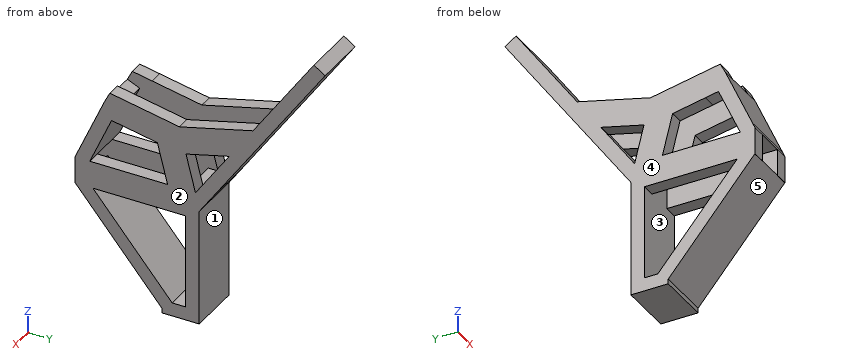
```python
from build123d import *

# Parameters (mm, degrees)
SKETCH_1_W       = 160
SKETCH_1_H       = 40
EXTRUDE_1_DEPTH  = 400
EXTRUDE_6_DEPTH  = 160
SKETCH_11_W      = 40
SKETCH_11_H      = 40
EXTRUDE_7_DEPTH  = 160
EXTRUDE_11_DEPTH = 160
SKETCH_17_W      = 40
SKETCH_17_H      = 80
EXTRUDE_13_DEPTH = 328
EXTRUDE_17_DEPTH = 160
EXTRUDE_18_DEPTH = 40
SKETCH_29_W      = 40
SKETCH_29_H      = 210
EXTRUDE_19_DEPTH = 80
EXTRUDE_20_DEPTH = 40
EXTRUDE_21_DEPTH = 40
EXTRUDE_22_DEPTH = 40


with BuildPart() as part:
    # Эскиз1 → Бобышка-Вытянуть1 (new body)
    with BuildSketch(Plane.XY):
        with Locations((41.709401709, 20)):
            Rectangle(SKETCH_1_W, SKETCH_1_H)
    extrude(amount=EXTRUDE_1_DEPTH)

    # Эскиз8 → Бобышка-Вытянуть6 (add)
    with BuildSketch(Plane.ZY.offset(38.290598291)):
        Polygon((403.40525509, 80.13918018), (346.080564925, 40), (400, 40), (400, 28.923811345), (901.472451167, 380.058601857), (878.529393713, 412.824683628), align=None)
    extrude(amount=-EXTRUDE_6_DEPTH)

    # Эскиз11 → Бобышка-Вытянуть7 (add)
    with BuildSketch(Plane.ZY.offset(38.290598291)):
        with Locations((20, -20)):
            Rectangle(SKETCH_11_W, SKETCH_11_H)
    extrude(amount=-EXTRUDE_7_DEPTH)

    # Эскиз12 → Бобышка-Вытянуть11 (add)
    with BuildSketch(Plane.ZY.offset(38.290598291)):
        Polygon((346.417777248, -297.115043875), (40, -40), (0, -40), (0, -70.641777725), (14.288495613, -70.641777725), (320.70627286, -327.756821599), align=None)
    extrude(amount=-EXTRUDE_11_DEPTH)

    # Эскиз17 → Бобышка-Вытянуть13 (add)
    with BuildSketch(Plane(origin=(0, 0, 0), x_dir=(-1, 0, 0), z_dir=(0, -1, 0))):
        with Locations((18.290598291, -360)):
            Rectangle(SKETCH_17_W, SKETCH_17_H)
        with Locations((-101.709401709, -360)):
            Rectangle(SKETCH_17_W, SKETCH_17_H)
    extrude(amount=EXTRUDE_13_DEPTH)

    # Эскиз26 → Бобышка-Вытянуть17 (add)
    with BuildSketch(Plane.ZY.offset(38.290598291)):
        Polygon((400, -284.21454886), (400, -328), (416.269465723, -320.756367165), align=None)
        Polygon((582.709091529, -202.867220245), (598.978557252, -239.40903855), (416.269465723, -320.756367165), (400, -284.21454886), align=None)
    extrude(amount=-EXTRUDE_17_DEPTH)

    # Эскиз27 → Бобышка-Вытянуть18 (add)
    with BuildSketch(Plane.ZY.offset(38.290598291)):
        Polygon((509.482462661, -33.639974138), (588.04709667, -18.55361331), (616.334023223, -165.862302077), (537.769389214, -180.948662905), align=None)
        Polygon((545.18630579, -219.573440808), (582.709091529, -202.867220245), (595.238756951, -231.009309548), (627.648793843, -224.785777584), (616.334023223, -165.862302077), (537.769389214, -180.948662905), align=None)
        Polygon((627.648793843, -224.785777584), (595.238756951, -231.009309548), (598.978557252, -239.40903855), align=None)
    extrude(amount=-EXTRUDE_18_DEPTH)

    # Эскиз29 → Бобышка-Вытянуть19 (add)
    with BuildSketch(Plane(origin=(0, 108.244163778, 563.698774535), x_dir=(1, 0, 0), z_dir=(0, 0.18857951034822912, 0.9820579251127819))):
        with Locations((101.709401709, -234.114356543)):
            Rectangle(SKETCH_29_W, SKETCH_29_H)
    extrude(amount=-EXTRUDE_19_DEPTH)

    # Эскиз33 → Бобышка-Вытянуть20 (add)
    with BuildSketch(Plane(origin=(121.709401709, 0, 0), x_dir=(0, 0, -1), z_dir=(1, 0, 0))):
        Polygon((-627.648793843, -224.785777584), (-598.978557252, -239.40903855), (-595.238756951, -231.009309548), align=None)
    extrude(amount=-EXTRUDE_20_DEPTH)

    # Эскиз34 → Бобышка-Вытянуть21 (add)
    with BuildSketch(Plane.ZY.offset(38.290598291)):
        Polygon((400, -53.586571178), (490.897529352, -76.536037974), (510.481100679, 1.029958017), (400, 28.923811345), align=None)
        Polygon((510.481100679, 1.029958017), (490.897529352, -76.536037974), (514.961644961, -62.173691245), (509.482462661, -33.639974138), (588.04709667, -18.55361331), align=None)
        Polygon((514.961644961, -62.173691245), (490.897529352, -76.536037974), (519.0862075, -83.653009555), align=None)
        Polygon((542.761910091, 128.886776961), (510.481100679, 1.029958017), (588.04709667, -18.55361331), (642.991448698, 199.068255444), align=None)
    extrude(amount=-EXTRUDE_21_DEPTH)

    # Эскиз35 → Бобышка-Вытянуть22 (add)
    with BuildSketch(Plane(origin=(121.709401709, 0, 0), x_dir=(0, 0, -1), z_dir=(1, 0, 0))):
        Polygon((-588.04709667, -18.55361331), (-643.423626769, 199.370869787), (-543.015704436, 129.064485674), (-510.437956524, 0.860554126), (-400, 28.923811345), (-400, -53.618639699), (-519.131929063, -83.891111895), (-509.482462661, -33.639974138), align=None)
    extrude(amount=-EXTRUDE_22_DEPTH)


solid = part.part
```
Could you check a few things on this model? Use its own coordinates, in mm. Face numbers are marked on the shaded views. A direction names the side the tool comes from. Round coordinates to 2 decimals unless told otherwise and drop trailing zeros. Order: outer loops, then holes, each group sorted by start corner. A loop starts at its lowest first (then second) coordinate and runs counter-clockwise, first axis right, second up. Notation, with made-up numbers: M 70,54 L 129,54 A28 ccw 129,93 Z; hole C 54.5,36 d10. An arc over 180 degrees is marked long. One line per question, with ' | ' between items. Start each with the question number.
(1) For the marked faces 1 and 2, which set-ups out of +Z, -Z, +X, -X, +Y, -Y let a thin tool reach every point of the face, with its end or its side?
(2) Suppose I cut it at B-B on x = -10. List the corners of the cut face in (y, z) for me, then the cut area to 3 significant figures.
(3) Suppose I cut it at A-A on x = 64. List the corners of the cut face in (y, z) for me.
(4) Suppose I cut it at C-C on y = 117. List the corners of the cut face in (x, z) for me, then the cut area to 3 significant figures.
(5) Please list where these lines run through material, in increasing order: line 1 along Z through (x, y) = (87, -191); line 2 along Z through (x, y) = (-31, -139); line 3 along Y through (x, z) = (-8, 212.5).
(6) Thinking about a two-plate mould opening in Z: for the marked faces 3, 4 and 5, which applies, +Z half, -Z half, draft (parallel to the pull), parting line (faces both ways), or undercut?
(7) For P1, Ø7, axis at x = 76.5, z = 8.5, coming from the -Y side; P2, Ø4, axis at x = 9.5, z = 431, coming from the +Y side; P3, Ø12, axis at x = 36, y = -19, coming from the +Z side, each with a flat end and sliding along its axis, tell me the tip position at first contact or that it passes through.
(8) Suppose I cut it at D-D on z = 80. List the corners of the cut face in (x, y) for me, then the cut area to 3 significant figures.
Geometry results:
1) face 1: -Z, +X, -X, +Y | face 2: +Z, -Z, +X, +Y, -Y
2) outline: M -328,320 L -327.16,320 L -70.64,14.29 L -70.64,0 L 40,0 L 40,346.08 L 412.82,878.53 L 380.06,901.47 L 199.07,642.99 L -18.55,588.05 L -224.79,627.65 L -239.41,598.98 L -328,400 Z; hole M -284.21,400 L -53.59,400 L -83.65,519.09 L -219.57,545.19 Z; hole M -274.95,320 L -40,40 L 0,40 L 0,320 Z; hole M 1.03,510.48 L 28.92,400 L 128.89,542.76 Z | area: 134,000 mm²
3) outline: M -328,400 L -284.21,400 L -202.87,582.71 L -239.41,598.98 Z; M -327.76,320.71 L -70.64,14.29 L -70.64,0 L 40,0 L 40,346.08 L 412.82,878.53 L 380.06,901.47 L 28.92,400 L 0,400 L 0,40 L -40,40 L -297.12,346.42 Z
4) outline: M -38.29,456.05 L 121.71,456.05 L 121.71,525.79 L -38.29,525.79 Z; M -38.29,539.76 L 1.71,539.76 L 1.71,622.27 L -38.29,622.27 Z; M 81.71,539.95 L 121.71,539.95 L 121.71,622.49 L 81.71,622.49 Z | area: 17,800 mm²
5) line 1: 157.73 to 219.95, 320 to 400, 539.7 to 621.16 | line 2: 95.75 to 157.98, 320 to 400, 529.71 to 611.18 | line 3: -236.96 to -184.74, 0 to 40
6) face 3: undercut | face 4: draft | face 5: -Z half
7) P1: y = -70.64 | P2: y = 100.86 | P3: z = 40
8) outline: M -38.29,-125.78 L 121.71,-125.78 L 121.71,-73.56 L -38.29,-73.56 Z; M -38.29,0 L 121.71,0 L 121.71,40 L -38.29,40 Z | area: 14,800 mm²
